Geometry check sheet. Reference: the model listing, model coordinates, mm. A direction names the side the tool comes from. Coordinates: 2 decimals unless noted, no trailing zeros. Order: outer loops, then holes, each group sorted by start corner. A loop starts at its lowest first (then second) coordinate and runs counter-clockwise, first axis right, second up. Notation, with made-up numbers: (34, 61.5) - (48, 61.5) arc R14 cw to (48, 83.5) - close; hole circle Ø11 at (28.25, 19). An arc over 180 degrees is marked (long way). Put each result on its own line as item: value.
from build123d import *

# Parameters (mm, degrees)
F0_R     = 6
F0_R_2   = 2.5
F1_DEPTH = 10
F3_R     = 7
F3_R_2   = 4.84
F4_DEPTH = 11


with BuildPart() as f1:
    # F0 (on Front) → F1 (new body, symmetric)
    with BuildSketch(Plane.XZ):
        Circle(F0_R)
        Circle(F0_R_2, mode=Mode.SUBTRACT)
    extrude(amount=F1_DEPTH, both=True)

    # F3 (on offset) → F4 (cut)
    with BuildSketch(Plane.XZ.offset(9)):
        Circle(F3_R)
        Circle(F3_R_2, mode=Mode.SUBTRACT)
    extrude(amount=-F4_DEPTH, mode=Mode.SUBTRACT)


solid = f1.part
Q1. Draft check along Y on faces 1 (the cylindrical face through (-0.54, 0.14, -2.44)), 2 (the flat face through (3, 10, 0)), 3 (the flat face through (-4, -9, 3)), 4 (the flat face through (3, -10, 0)). Enter one of: pulls with the +Y half, pulls with the -Y half, needs draft (parallel to the pull), parting line crosses it, or undercut.
Answer block:
face 1: needs draft
face 2: pulls with the +Y half
face 3: undercut
face 4: pulls with the -Y half
Q2. Access from +Z, -Z, +X, -X, +Y, -Y to the whole of each face (thin tool, end or side, straight path). Record for faces 5 (the cylindrical face through (-5.994, -9.507, 0.264)), 6 (the flat face through (-4, 2, 3)).
Answer block:
face 5: +Y, -Y
face 6: none
Q3. Depth check by flat-ended pin: pin 1 Ø1 at (y, z) = (-1, 3.5) entering from -X; pin 2 Ø5 at (y, z) = (-7, -2) entering from +X; pin 3 Ø3 at (y, z) = (2, 3) entering from +X. Enter the tip coordinate at first touch or a pass-through.
Answer block:
pin 1: stops at x = -3.8
pin 2: stops at x = 5.98
pin 3: stops at x = 5.81
Q4. Section check D-D on z = 4.5. Record the boundary of the cut face in (x, y), then the cut area to 3 significant figures.
Answer block:
outline: (-3.97, -10) - (3.97, -10) - (3.97, -9) - (1.78, -9) - (1.78, 2) - (3.97, 2) - (3.97, 10) - (-3.97, 10) - (-3.97, 2) - (-1.78, 2) - (-1.78, -9) - (-3.97, -9) - close
area: 111 mm^2
Q5. Section check A-A on x = 0. Record the boundary of the cut face in (y, z).
Answer block:
outline: (-10, -6) - (-9, -6) - (-9, -4.84) - (2, -4.84) - (2, -6) - (10, -6) - (10, -2.5) - (-10, -2.5) - close; (-10, 2.5) - (10, 2.5) - (10, 6) - (2, 6) - (2, 4.84) - (-9, 4.84) - (-9, 6) - (-10, 6) - close
Q6. Section check B-B on z = -1.75. Record the boundary of the cut face in (x, y), then the cut area to 3 significant figures.
Answer block:
outline: (-5.74, -10) - (-1.79, -10) - (-1.79, 10) - (-5.74, 10) - (-5.74, 2) - (-4.51, 2) - (-4.51, -9) - (-5.74, -9) - close; (1.79, -10) - (5.74, -10) - (5.74, -9) - (4.51, -9) - (4.51, 2) - (5.74, 2) - (5.74, 10) - (1.79, 10) - close
area: 131 mm^2
Q7. Thickness scan on L1, parallel to Z at x = 0, y = 4.75; L2, parallel to Y at x = 4.5, z = -3; L3, parallel to Z at x = 0, y = -4.25. Record the ranges inside material, lowest first. Write a range as [from, to].
Answer block:
L1: z = [-6, -2.5], [2.5, 6]
L2: y = [-10, -9], [2, 10]
L3: z = [-4.84, -2.5], [2.5, 4.84]
Q8. Section check C-C on y = -1.25. Record the boundary of the cut face in (x, z), then the cut area to 3 significant figures.
Answer block:
outline: circle Ø9.68 at (0, 0); hole circle Ø5 at (0, 0)
area: 54.0 mm^2
